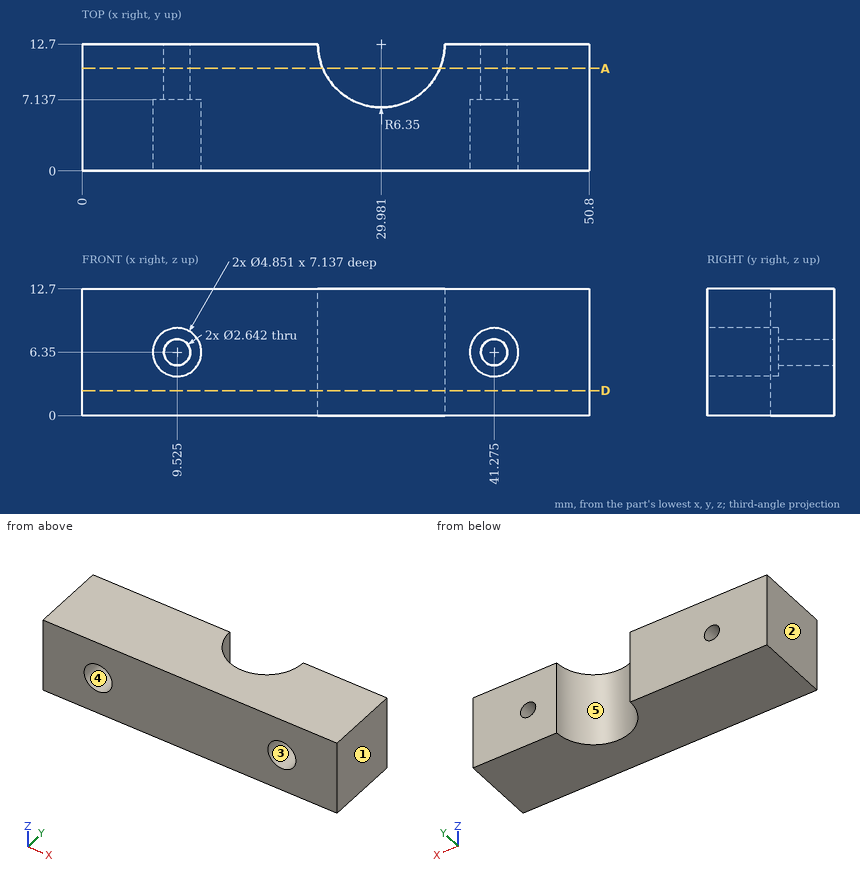
Source: three-view drawing plus pictorial views. Frame: mm from the lowest corner of the part. A direction names the side the tool comes from. Give positions to 0.01 mm unless a question says otherwise; leave off trailing zeros. Write each loop counter-clockwise with the first axis right and the second up, starting at its lowest first coordinate (ties: lowest second). Pieces come first, ordered by that corner, then holes. Notation, with made-up numbers: (-30.75, 2.5) -> (-10.75, 2.5) arc R31 cw to (-10.75, 32.5) -> close; hole circle Ø2 at (88.5, 28.25). An arc over 180 degrees is marked (long way). Write item = value, one per line.
Q1. Cut plane D-D on z = 2.5. Return loops of the section in (x, y), then the cut area to 3 significant figures.
Here are the results:
outline = (0, 0) -> (50.8, 0) -> (50.8, 12.7) -> (36.33, 12.7) arc R6.35 cw to (23.63, 12.7) -> (0, 12.7) -> close
area = 582 mm²
Q2. Line query: line 1 (X direction, y = 5.75, z = 6.25); line 2 (X direction, y = 11.3, z = 6.35) (1 decimal); line 3 (X direction, y = 10.25, z = 6.35) (1 decimal). Output: solid intervals per line, ascending. Write a range as from..to.
Here are the results:
line_1 = 0..7.1, 11.95..38.85, 43.7..50.8
line_2 = 0..8.2, 10.8..23.8, 36.2..40, 42.6..50.8
line_3 = 0..8.2, 10.8..24.1, 35.8..40, 42.6..50.8
Q3. Reachability of the marked faces 4 and 5 from +Z, -Z, +X, -X, +Y, -Y: full face, straight path, thin tool, end or side. Return the list, or none.
Here are the results:
face_4 = -Y
face_5 = +Z, -Z, +Y
Q4. Mould query, pull axis X, two halves, no side actions, for the marked faces 1, 2 and 3. Classes: +X half, -X half, draft (parallel to the pull), parting line (faces both ways), or undercut.
Here are the results:
face_1 = +X half
face_2 = -X half
face_3 = undercut
Q5. Cut plane A-A on y = 10.25. State how many separate pieces and enclosed holes the cut face has.
Here are the results:
separate_pieces = 2
enclosed_holes = 2
